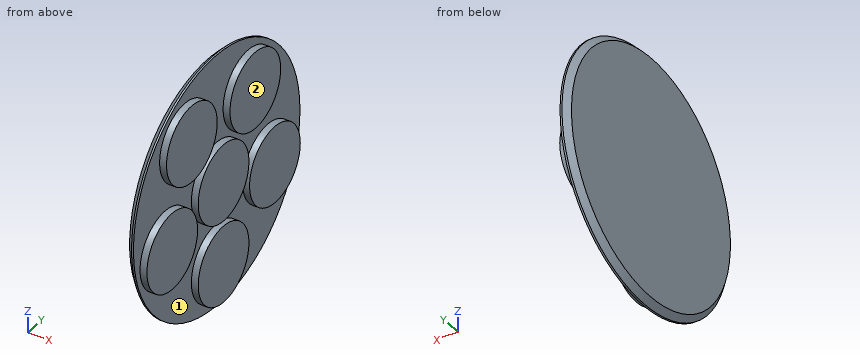
from build123d import *

# Parameters (mm, degrees)
F0_R     = 16.5
F1_DEPTH = 1
F2_R     = 5.025
F3_DEPTH = 0.9
F4_SIZE  = 0.75


with BuildPart() as f1:
    # F0 (on Right) → F1 (new body)
    with BuildSketch(Plane.YZ):
        Circle(F0_R)
    extrude(amount=F1_DEPTH)

    # F2 (on face) → F3 (join)
    with BuildSketch(Plane.YZ.offset(1)):
        Circle(F2_R)
        with Locations((0, -10.7)):
            Circle(F2_R)
        with Locations((10.176305, -3.306482)):
            Circle(F2_R)
        with Locations((6.289302, 8.656482)):
            Circle(F2_R)
        with Locations((-6.289302, 8.656482)):
            Circle(F2_R)
        with Locations((-10.176305, -3.306482)):
            Circle(F2_R)
    extrude(amount=F3_DEPTH)

    # F4
    f4_edges = [f1.edges().sort_by_distance(p)[0] for p in [
        (0, -16.5, 0),
    ]]
    chamfer(f4_edges, length=F4_SIZE)


solid = f1.part
Check sheet for the modelled part. Datum: model origin and axes. Units: mm. Face numbers are marked on the shaded views. Round coordinates to 2 decimals unless told otherwise and drop trailing zeros. Order: outer loops, then holes, each group sorted by start corner. A loop starts at its lowest first (then second) coordinate and runs counter-clockwise, first axis right, second up.
(1) Cross-section at C-C, the plane x = 1.4. Enter the section's corners in (y, z) (3 decimals).
(2) Cross-section at A-A, the plane y = 0. Enter the section's corners in (x, z) (3 decimals).
(3) Go/stop test with a flat-tipped pin: P1, Ø1, axis at x = 0.5, z = -5, coming from the -Y side. Record where the tip stops, or that it passes through.
(4) Draft check along Z on the marked faces 1 and 2. Enter one of: pulls with the +Z half, pulls with the -Z half, needs draft (parallel to the pull), parting line crosses it, or undercut.
(5) Cross-section at B-B, the plane z = 0. Enter the section's corners in (x, y) (3 decimals), and give its area (3 significant figures).
(6) Scan lines: probe 1 along Z at (x, y) = (1.25, -4.5); probe 2 along Z at (x, y) = (1.7, 0) (3 decimals); probe 3 along Y at (x, z) = (1.15, 12). Record each from-to range of solid material in increasing order.
Check sheet entries:
1. outline: circle Ø10.05 at (-10.176, -3.306); circle Ø10.05 at (-6.289, 8.656); circle Ø10.05 at (0, -10.7); circle Ø10.05 at (0, 0); circle Ø10.05 at (6.289, 8.656); circle Ø10.05 at (10.176, -3.306)
2. outline: (0, -15.75) - (0.75, -16.5) - (1, -16.5) - (1, -15.725) - (1.9, -15.725) - (1.9, -5.675) - (1, -5.675) - (1, -5.025) - (1.9, -5.025) - (1.9, 5.025) - (1, 5.025) - (1, 16.5) - (0.75, 16.5) - (0, 15.75) - close
3. P1: stops at y = -15.86
4. face 1: undercut
4. face 2: needs draft
5. outline: (0, -15.75) - (0.75, -16.5) - (1, -16.5) - (1, -13.96) - (1.9, -13.96) - (1.9, -6.392) - (1, -6.392) - (1, -5.025) - (1.9, -5.025) - (1.9, 5.025) - (1, 5.025) - (1, 6.392) - (1.9, 6.392) - (1.9, 13.96) - (1, 13.96) - (1, 16.5) - (0.75, 16.5) - (0, 15.75) - close
5. area: 55.1 mm2
6. probe 1: z = -12.94 to -8.46, -2.24 to 2.24, 3.96 to 13.35
6. probe 2: z = -15.725 to -5.675, -5.025 to 5.025
6. probe 3: y = -10.04 to -2.54, 2.54 to 10.04
